```python
from build123d import *

# Parameters (mm, degrees)
BOSS_EXTRUDE1_DEPTH = 3.175
CUT_EXTRUDE1_DEPTH  = 3.175


with BuildPart() as part:
    # Sketch1 → Boss-Extrude1 (new body)
    with BuildSketch(Plane.XY):
        with BuildLine():
            ThreePointArc((-3.882285677, 14.488887394), (-1.685586535, 12.803300859), (0, 15))
            ThreePointArc((0, 15), (2.196699141, 16.685586535), (3.882285677, 14.488887394))
            ThreePointArc((3.882285677, 14.488887394), (4.941889669, 11.930777064), (7.5, 12.990381057))
            ThreePointArc((7.5, 12.990381057), (10.245190528, 13.351792246), (10.606601718, 10.606601718))
            ThreePointArc((10.606601718, 10.606601718), (10.245190528, 7.861411189), (12.990381057, 7.5))
            ThreePointArc((12.990381057, 7.5), (15.548491387, 6.440396007), (14.488887394, 3.882285677))
            ThreePointArc((14.488887394, 3.882285677), (12.803300859, 1.685586535), (15, 0))
            ThreePointArc((15, 0), (16.685586535, -2.196699141), (14.488887394, -3.882285677))
            ThreePointArc((14.488887394, -3.882285677), (11.930777064, -4.941889669), (12.990381057, -7.5))
            ThreePointArc((12.990381057, -7.5), (13.351792246, -10.245190528), (10.606601718, -10.606601718))
            ThreePointArc((10.606601718, -10.606601718), (7.861411189, -10.245190528), (7.5, -12.990381057))
            ThreePointArc((7.5, -12.990381057), (6.440396007, -15.548491387), (3.882285677, -14.488887394))
            ThreePointArc((3.882285677, -14.488887394), (1.685586535, -12.803300859), (0, -15))
            ThreePointArc((0, -15), (-2.196699141, -16.685586535), (-3.882285677, -14.488887394))
            ThreePointArc((-3.882285677, -14.488887394), (-4.941889669, -11.930777064), (-7.5, -12.990381057))
            ThreePointArc((-7.5, -12.990381057), (-10.245190528, -13.351792246), (-10.606601718, -10.606601718))
            ThreePointArc((-10.606601718, -10.606601718), (-10.245190528, -7.861411189), (-12.990381057, -7.5))
            ThreePointArc((-12.990381057, -7.5), (-15.548491387, -6.440396007), (-14.488887394, -3.882285677))
            ThreePointArc((-14.488887394, -3.882285677), (-12.803300859, -1.685586535), (-15, 0))
            ThreePointArc((-15, 0), (-16.685586535, 2.196699141), (-14.488887394, 3.882285677))
            ThreePointArc((-14.488887394, 3.882285677), (-11.930777064, 4.941889669), (-12.990381057, 7.5))
            ThreePointArc((-12.990381057, 7.5), (-13.351792246, 10.245190528), (-10.606601718, 10.606601718))
            ThreePointArc((-10.606601718, 10.606601718), (-7.861411189, 10.245190528), (-7.5, 12.990381057))
            ThreePointArc((-7.5, 12.990381057), (-6.440396007, 15.548491387), (-3.882285677, 14.488887394))
        make_face()
    extrude(amount=BOSS_EXTRUDE1_DEPTH)

    # Sketch3 → Cut-Extrude1 (cut)
    with BuildSketch(Plane.XY):
        Polygon((3.231601359, 12.384139409), (0.083763924, 12.79856007), (-3.231601359, -12.384139409), (-0.083763924, -12.79856007), align=None)
    extrude(amount=CUT_EXTRUDE1_DEPTH, mode=Mode.SUBTRACT)


solid = part.part
```
The model under review builds one solid part; all positions refer to its coordinate system, in mm. A direction names the side the tool comes from. Round coordinates to 2 decimals unless told otherwise and drop trailing zeros. Loops run counter-clockwise (first coordinate to the right, second up) from the corner with the lowest first, then second, coordinate; pieces in that order, holes last. Notation, with made-up numbers: (-14, -18) -> (1, -18) arc R37 cw to (1, 18) -> close; hole circle Ø3 at (83, 41). An arc over 180 degrees is marked (long way). Answer in a Markdown table with one row per item.
1) Consider section A-A, the plane z = 2.3. Write out the cut boundary in (x, y), plus the area to 3 significant figures.
Taken from the geometry:
| item | result |
|---|---|
| outline | (-15, 0) arc R1.96 cw to (-14.49, -3.88) arc R1.96 ccw to (-12.99, -7.5) arc R1.96 cw to (-10.61, -10.61) arc R1.96 ccw to (-7.5, -12.99) arc R1.96 cw to (-3.88, -14.49) arc R1.96 ccw to (0, -15) arc R1.96 cw to (3.88, -14.49) arc R1.96 ccw to (7.5, -12.99) arc R1.96 cw to (10.61, -10.61) arc R1.96 ccw to (12.99, -7.5) arc R1.96 cw to (14.49, -3.88) arc R1.96 ccw to (15, 0) arc R1.96 cw to (14.49, 3.88) arc R1.96 ccw to (12.99, 7.5) arc R1.96 cw to (10.61, 10.61) arc R1.96 ccw to (7.5, 12.99) arc R1.96 cw to (3.88, 14.49) arc R1.96 ccw to (0, 15) arc R1.96 cw to (-3.88, 14.49) arc R1.96 ccw to (-7.5, 12.99) arc R1.96 cw to (-10.61, 10.61) arc R1.96 ccw to (-12.99, 7.5) arc R1.96 cw to (-14.49, 3.88) arc R1.96 ccw to start; hole (-3.23, -12.38) -> (-0.08, -12.8) -> (3.23, 12.38) -> (0.08, 12.8) -> close |
| area | 618 mm² |
2) For pin 1 Ø1 at (x, y) = (4, -2.5) entering from -Z, flat-tipped, find the tip position at first contact; note if it passes through.
Taken from the geometry:
| item | result |
|---|---|
| pin 1 | stops at z = 0 |
3) Wall thickness on line 1 along Y through (x, z) = (13, 1.2); line 2 along X through (y, z) = (10, 1.7); line 3 along X through (y, z) = (-14.5, 2.75): over which ranges is each line inside the solid? List them lowest first.
Taken from the geometry:
| item | result |
|---|---|
| line 1 | y = -10.6 to -7.51, -3.88 to 1.05, 2.83 to 7.5 |
| line 2 | x = -13.51 to -9.83, -8.28 to -0.28, 2.92 to 10.08 |
| line 3 | x = -3.88 to 0, 3.89 to 7.5 |
4) Consider section B-B, the plane y = 3. Write out the cut boundary in (x, z) (3 decimals).
Taken from the geometry:
| item | result |
|---|---|
| outline | (-16.391, 0) -> (-1.206, 0) -> (-1.206, 3.175) -> (-16.391, 3.175) -> close; (1.996, 0) -> (13.098, 0) -> (13.098, 3.175) -> (1.996, 3.175) -> close |
5) Consider section C-C, the plane y = 9. Write out the cut boundary in (x, z) (3 decimals), plus the area to 3 significant figures.
Taken from the geometry:
| item | result |
|---|---|
| outline | (-13.756, 0) -> (-0.416, 0) -> (-0.416, 3.175) -> (-13.756, 3.175) -> close; (2.786, 0) -> (9.841, 0) -> (9.841, 3.175) -> (2.786, 3.175) -> close |
| area | 64.8 mm² |
6) Tool access review of faces 4 (the flat face through (-3, 0, 0)), 5 (the flat face through (1.68, 12.59, 1.57)): name each direction out of +Z, -Z, +X, -X, +Y, -Y from which nothing blocks a thin tool from reaching the whole face with its end or side.
Taken from the geometry:
| item | result |
|---|---|
| face 4 | -Z, +X, -X, +Y, -Y |
| face 5 | +Z, -Z |
7) Draft analysis for pull direction X (two halves, no side actions). For faces 1 (the cylindrical face through (10.219, 7.896, 1.565)), 2 (the cylindrical face through (10.21, 13.38, 1.57)), 3 (the flat face through (-3, 0, 3.175)), state which applies: pulls with the +X half, pulls with the -X half, needs draft (parallel to the pull), parting line crosses it, or undercut.
Taken from the geometry:
| item | result |
|---|---|
| face 1 | undercut |
| face 2 | undercut |
| face 3 | needs draft |
8) Consider section D-D, the plane x = -8.5. Write out the cut boundary in (y, z) (3 decimals).
Taken from the geometry:
| item | result |
|---|---|
| outline | (-13.677, 0) -> (9.92, 0) -> (9.92, 3.175) -> (-13.677, 3.175) -> close |
